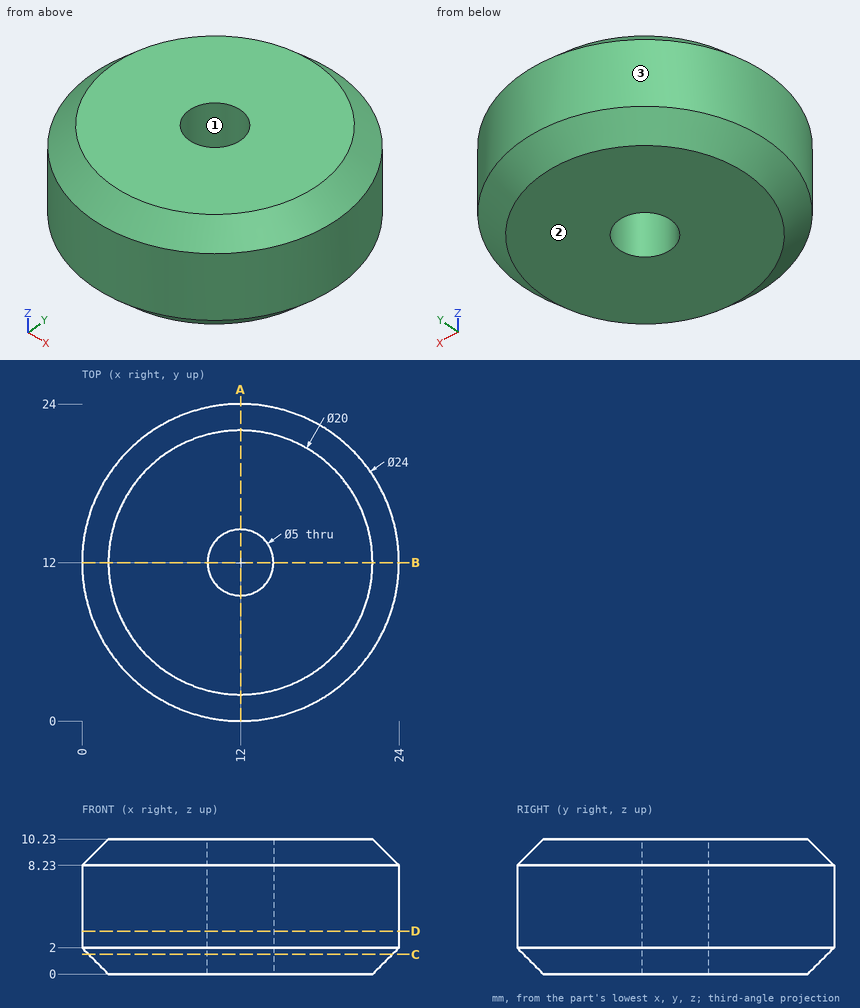
Part print with two shaded views. Sizes in mm from the minimum x, y, z corner. Coordinates: 2 decimals unless noted, no trailing zeros. Write each loop counter-clockwise with the first axis right and the second up, starting at its lowest first coordinate (ties: lowest second). Pieces come first, ordered by that corner, then holes.
1. Band-saw the part on C-C, the plane z = 1.5. Give the cut face in (x, y), and give its area (3 significant figures).
Answer block:
outline: circle Ø23 at (12, 12); hole circle Ø5 at (12, 12)
area: 396 mm2
2. Band-saw the part on D-D, the plane z = 3.25. Give the cut face in (x, y), and give its area (3 significant figures).
Answer block:
outline: circle Ø24 at (12, 12); hole circle Ø5 at (12, 12)
area: 433 mm2
3. Pull direction X, two halves, no side cores. Call the marked faces 1, 2 and 3: released by +X, released by -X, zero draft, split by the parting line, or undercut.
Answer block:
face 1: undercut
face 2: zero draft
face 3: split by the parting line
4. Drill centre lines: probe 1 along Y at (x, z) = (12, 5.5); probe 2 along Y at (x, z) = (13.5, 9.75); probe 3 along X at (y, z) = (13, 5.5). Where is each one in solid material? Low to high.
Answer block:
probe 1: y = 0 to 9.5, 14.5 to 24
probe 2: y = 1.63 to 10, 14 to 22.37
probe 3: x = 0.04 to 9.71, 14.29 to 23.96
5. Band-saw the part on A-A, the plane x = 12. Give the cut face in (y, z).
Answer block:
outline: (0, 2) - (2, 0) - (9.5, 0) - (9.5, 10.23) - (2, 10.23) - (0, 8.23) - close; (14.5, 0) - (22, 0) - (24, 2) - (24, 8.23) - (22, 10.23) - (14.5, 10.23) - close
6. Drop flat-ended pins along their axis: pin 1 (1 mm diameter, centred on x = 8, z = 4, fed in from +Y); pin 2 (2 mm diameter, centred on x = 10, z = 3, fed in from -Y); pin 3 (3 mm diameter, centred on x = 7, z = 1, fed in from +Y); pin 4 (4 mm diameter, centred on x = 12, y = 12, fed in from -Z). Give the stop position or say it passes through.
Answer block:
pin 1: stops at y = 23.48
pin 2: stops at y = 0.04
pin 3: stops at y = 23.35
pin 4: passes through
